Work out the finished part from the listing and answer in its coordinate system (mm). Face numbers are marked on the shaded views. A direction names the side the tool comes from. Give positions to 0.01 mm unless a question says otherwise; leave off trailing zeros. Order: outer loops, then holes, each group sorted by start corner. A loop starts at its lowest first (then second) coordinate and runs counter-clockwise, first axis right, second up. Notation, with made-up numbers: M -35.5,72.5 L -0.5,72.5 A25 cw -0.5,88.5 Z; hole C 74,-23 d9. An arc over 180 degrees is marked long. One line per item, written item: value.
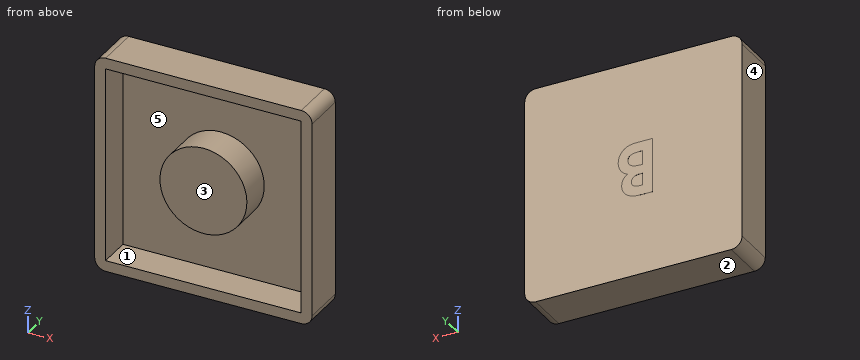
from build123d import *

# Parameters (mm, degrees)
SKETCH1_W           = 12.7
SKETCH1_H           = 12.7
BOSS_EXTRUDE1_DEPTH = 2.54
FILLET1_R           = 0.635
SHELL1_START        = 0.635
SHELL1_OUTLINE_W    = 1.905
SHELL1_OUTLINE_H    = 11.43
SHELL1_DEPTH        = 11.43
SKETCH2_R           = 2.54
BOSS_EXTRUDE2_DEPTH = 1.905
BOSS_EXTRUDE3_DEPTH = 0.00254


# Read off the part's stored shape, not the designer's step: Shell1
with BuildPart() as part:
    # Sketch1 → Boss-Extrude1 (new body)
    with BuildSketch(Plane(origin=(0, 0, 0), x_dir=(1, 0, 0), z_dir=(0, 1, 0))):
        with Locations((6.35, 6.35)):
            Rectangle(SKETCH1_W, SKETCH1_H)
    extrude(amount=BOSS_EXTRUDE1_DEPTH)

    # Fillet1
    fillet1_edges = [part.edges().sort_by_distance(p)[0] for p in [
        (0, 1.27, -12.7),
        (12.7, 1.27, -12.7),
        (12.7, 1.27, 0),
        (0, 1.27, 0),
    ]]
    fillet(fillet1_edges, radius=FILLET1_R)

    # Shell1 outline → Shell1 (cut)
    with BuildSketch(Plane.YZ.offset(SHELL1_START)):
        with Locations((0.9525, -6.35)):
            Rectangle(SHELL1_OUTLINE_W, SHELL1_OUTLINE_H)
    extrude(amount=SHELL1_DEPTH, mode=Mode.SUBTRACT)

    # Sketch2 → Boss-Extrude2 (add)
    with BuildSketch(Plane(origin=(0, 1.905, 0), x_dir=(-1, 0, 0), z_dir=(0, -1, 0))):
        with Locations(Location((-6.35, 6.35, 0), (0, 0, 270))):
            Circle(SKETCH2_R)
    extrude(amount=BOSS_EXTRUDE2_DEPTH)

    # Sketch3 → Boss-Extrude3 (add)
    with BuildSketch(Plane(origin=(0, 2.54, 0), x_dir=(1, 0, 0), z_dir=(0, 1, 0))):
        with BuildLine():
            Line((5.243146154, 4.826), (5.243146154, 8.001))
            Line((5.243146154, 8.001), (5.751960256, 8.001))
            add(Edge.make_bspline(
                [(5.751960256, 8.001), (5.787580425, 8.001004065), (5.856504776, 8.001011931), (5.955944627, 7.99751993), (6.048166691, 7.993002635), (6.132877481, 7.987948833), (6.210221182, 7.979240122), (6.280080178, 7.970062092), (6.34259405, 7.958993954), (6.381242981, 7.94906549), (6.399426202, 7.944394431)],
                knots=[0, 0, 0, 0, 1.311965854, 2.538629056, 3.664479157, 4.713267157, 5.663616078, 6.530575999, 7.308677837, 8, 8, 8, 8], degree=3))
            add(Edge.make_bspline(
                [(6.399426202, 7.944394431), (6.423302618, 7.937805819), (6.470155811, 7.924876846), (6.537264535, 7.898766227), (6.600926521, 7.869742423), (6.661064039, 7.836631691), (6.717307821, 7.799034291), (6.769444122, 7.75665184), (6.818597392, 7.711185567), (6.863022312, 7.66136834), (6.903175119, 7.608727211), (6.93806071, 7.553275975), (6.968371817, 7.495862516), (6.992628642, 7.435764324), (7.010905704, 7.373258168), (7.02427347, 7.308610959), (7.032937594, 7.241618137), (7.03375624, 7.19604073), (7.034171795, 7.172905048)],
                knots=[0, 0, 0, 0, 1.099996261, 2.158545794, 3.195537121, 4.207578794, 5.205712374, 6.197378256, 7.190519799, 8.17788031, 9.159561366, 10.129234751, 11.085776129, 12.040971148, 13.00380137, 13.975669004, 14.972423361, 16, 16, 16, 16], degree=3))
            add(Edge.make_bspline(
                [(7.034171795, 7.172905048), (7.033085241, 7.143181769), (7.030946494, 7.084675147), (7.01728403, 6.998739505), (6.99166478, 6.917517971), (6.958142616, 6.839513663), (6.912562953, 6.765017538), (6.854685596, 6.694065017), (6.785447969, 6.624471365), (6.732338887, 6.582754665), (6.704714663, 6.56105609)],
                knots=[0, 0, 0, 0, 0.986156485, 1.941127874, 2.875419072, 3.804401753, 4.751181392, 5.761612777, 6.835722519, 8, 8, 8, 8], degree=3))
            add(Edge.make_bspline(
                [(6.704714663, 6.56105609), (6.727100009, 6.549628565), (6.770991478, 6.527222351), (6.833304469, 6.490393223), (6.890999497, 6.451220775), (6.944335248, 6.410493172), (6.992192945, 6.366483912), (7.036548712, 6.321728868), (7.075214265, 6.273663764), (7.109790168, 6.22400173), (7.139842981, 6.172023655), (7.166015667, 6.117817318), (7.188122796, 6.061197538), (7.206843685, 6.002452465), (7.220805729, 5.941380042), (7.229909278, 5.877958428), (7.236879525, 5.812403923), (7.237421744, 5.76774983), (7.237697436, 5.745045473)],
                knots=[0, 0, 0, 0, 1.164658916, 2.283573913, 3.35186032, 4.395461096, 5.390182219, 6.362969632, 7.312859996, 8.245001507, 9.165155236, 10.092416118, 11.032087915, 11.979892451, 12.947605196, 13.931445124, 14.948243989, 16, 16, 16, 16], degree=3))
            add(Edge.make_bspline(
                [(7.237697436, 5.745045473), (7.235908383, 5.701681448), (7.232377694, 5.616102718), (7.20656302, 5.490453489), (7.161808578, 5.371326623), (7.101712592, 5.259195582), (7.027662773, 5.157306375), (6.942526717, 5.068052315), (6.847161548, 4.992500734), (6.759175654, 4.941509278), (6.683074784, 4.907289243), (6.620041855, 4.886132259), (6.552345826, 4.866532461), (6.478746667, 4.852769079), (6.400578631, 4.840171317), (6.317079575, 4.832393198), (6.228405558, 4.827122159), (6.167500409, 4.826381615), (6.136114904, 4.826)],
                knots=[0, 0, 0, 0, 1.284142165, 2.534249414, 3.780121997, 5.041676246, 6.291546858, 7.49970053, 8.684500223, 9.883330709, 10.50184324, 11.153274765, 11.851151195, 12.587658647, 13.369265475, 14.195992086, 15.070362669, 16, 16, 16, 16], degree=3))
            Line((6.136114904, 4.826), (5.243146154, 4.826))
        make_face()
        with BuildLine():
            Line((5.813017949, 7.431128205), (5.813017949, 6.739141026))
            Line((5.813017949, 6.739141026), (5.964390144, 6.739141026))
            add(Edge.make_bspline(
                [(5.964390144, 6.739141026), (5.984962986, 6.739320429), (6.024677611, 6.739666755), (6.082041174, 6.744127321), (6.135380025, 6.751737323), (6.184491859, 6.762355191), (6.229834171, 6.775838335), (6.271117303, 6.792061461), (6.308159738, 6.811855437), (6.351194481, 6.841339439), (6.396685308, 6.884726468), (6.436730371, 6.94740802), (6.460316645, 7.019491567), (6.46294352, 7.070330466), (6.4643, 7.096582933)],
                knots=[0, 0, 0, 0, 1.065314748, 2.056525647, 2.977365736, 3.853934255, 4.656397591, 5.425096493, 6.14721249, 6.826394842, 8.123232004, 9.372140726, 10.643011755, 12, 12, 12, 12], degree=3))
            add(Edge.make_bspline(
                [(6.4643, 7.096582933), (6.463214568, 7.12117273), (6.461115928, 7.168716114), (6.437367582, 7.235471259), (6.400481706, 7.29462998), (6.356932744, 7.335119286), (6.315922935, 7.362772289), (6.280807819, 7.380980614), (6.242266343, 7.39728052), (6.199552384, 7.409743825), (6.152909864, 7.419095851), (6.10256535, 7.425963794), (6.048431981, 7.430638408), (6.011041948, 7.430961437), (5.991738902, 7.431128205)],
                knots=[0, 0, 0, 0, 1.347982417, 2.606269829, 3.849316587, 5.153353503, 5.842674298, 6.568177932, 7.326619318, 8.142485038, 9.012069166, 9.942760135, 10.937925643, 12, 12, 12, 12], degree=3))
            Line((5.991738902, 7.431128205), (5.813017949, 7.431128205))
        make_face(mode=Mode.SUBTRACT)
        with BuildLine():
            Line((5.813017949, 6.209974359), (5.813017949, 5.395871795))
            Line((5.813017949, 5.395871795), (5.977110497, 5.395871795))
            add(Edge.make_bspline(
                [(5.977110497, 5.395871795), (6.009551802, 5.396057131), (6.071924261, 5.396413462), (6.161272697, 5.400718795), (6.242512762, 5.408478398), (6.315429202, 5.418165637), (6.3801337, 5.431290331), (6.436407542, 5.447976697), (6.485022448, 5.466334606), (6.525686923, 5.489008804), (6.558907469, 5.515395947), (6.588885529, 5.542364242), (6.613327771, 5.573474717), (6.632666929, 5.607391887), (6.649404936, 5.643273225), (6.65950012, 5.682519883), (6.667186238, 5.723968686), (6.667609226, 5.752637926), (6.667825641, 5.76730609)],
                knots=[0, 0, 0, 0, 1.753078804, 3.370512758, 4.83203934, 6.162291463, 7.344201807, 8.395507345, 9.331626367, 10.147333109, 10.898971645, 11.62040215, 12.321813352, 13.025280112, 13.727906689, 14.453419512, 15.208716525, 16, 16, 16, 16], degree=3))
            add(Edge.make_bspline(
                [(6.667825641, 5.76730609), (6.667348384, 5.784079366), (6.666418815, 5.816749196), (6.658827018, 5.864499638), (6.645030243, 5.909077845), (6.627652532, 5.95162374), (6.603470524, 5.990614032), (6.574731033, 6.027398029), (6.540006391, 6.060730109), (6.500956506, 6.092626322), (6.455408681, 6.120553184), (6.403341547, 6.144784684), (6.344472246, 6.165021941), (6.278618424, 6.181134857), (6.206068781, 6.194809667), (6.126293782, 6.202975038), (6.039957822, 6.209047983), (5.980091063, 6.209658551), (5.949125721, 6.209974359)],
                knots=[0, 0, 0, 0, 0.845221588, 1.646264278, 2.427170338, 3.19324141, 3.95557735, 4.731569926, 5.540061037, 6.376114724, 7.268642756, 8.224665384, 9.265483498, 10.400594375, 11.639216012, 12.983232105, 14.439614077, 16, 16, 16, 16], degree=3))
            Line((5.949125721, 6.209974359), (5.813017949, 6.209974359))
        make_face(mode=Mode.SUBTRACT)
    extrude(amount=BOSS_EXTRUDE3_DEPTH)


solid = part.part
(1) Section B-B, the plane z = -9.75 is taken. Give the vertices of the cut face in (x, y) (3 decimals), then the cut area to 3 significant figures.
Findings:
outline: M 0,0 L 0.635,0 L 0.635,1.905 L 12.065,1.905 L 12.065,0 L 12.7,0 L 12.7,2.54 L 0,2.54 Z
area: 10.5 mm^2
(2) Find the intervals of material crossed by probe 1 along Z at (x, y) = (6.5, 0.55) (3 decimals); probe 2 along Z at (x, y) = (11, 1.2) (3 decimals); probe 3 along X at (y, z) = (0.8, -5) (3 decimals), in increasing order. Write a range as from..to.
Findings:
probe 1: z = -12.7..-12.065, -8.886..-3.814, -0.635..0
probe 2: z = -12.7..-12.065, -0.635..0
probe 3: x = 0..0.635, 4.198..8.502, 12.065..12.7
(3) Section C-C, the plane x = 2.25 is taken. Give the vertices of the cut face in (y, z) (3 decimals), then the cut area to 3 significant figures.
Findings:
outline: M 0,-12.7 L 2.54,-12.7 L 2.54,0 L 0,0 L 0,-0.635 L 1.905,-0.635 L 1.905,-12.065 L 0,-12.065 Z
area: 10.5 mm^2
(4) Section D-D, the plane x = 4.25 is taken. Give the vertices of the cut face in (y, z) (3 decimals), then the cut area to 3 significant figures.
Findings:
outline: M 0,-12.7 L 2.54,-12.7 L 2.54,0 L 0,0 L 0,-0.635 L 1.905,-0.635 L 1.905,-4.921 L 0,-4.921 L 0,-7.779 L 1.905,-7.779 L 1.905,-12.065 L 0,-12.065 Z
area: 15.9 mm^2
(5) Section A-A, the plane y = 1.1 is taken. Give the vertices of the cut face in (x, z) (3 decimals), then the cut area to 3 significant figures.
Findings:
outline: M 0,-12.065 A0.635 ccw 0.635,-12.7 L 12.065,-12.7 A0.635 ccw 12.7,-12.065 L 12.7,-0.635 A0.635 ccw 12.065,0 L 0.635,0 A0.635 ccw 0,-0.635 Z; C 6.35,-6.35 d5.08; hole M 0.635,-12.065 L 12.065,-12.065 L 12.065,-0.635 L 0.635,-0.635 Z
area: 50.6 mm^2
(6) Which of the six approach directions +Z, -Z, +X, -X, +Y, -Y give full straight-line access (tool end or side, diameter ignored) to the marked faces 4 and 5?
Findings:
face 4: +Z, -Z, -X, +Y, -Y
face 5: -Y
(7) Determine the mould class of the marked faces 1, 2 and 3 for opening direction Z: pulls with the +Z half, pulls with the -Z half, needs draft (parallel to the pull), parting line crosses it, or undercut.
Findings:
face 1: undercut
face 2: pulls with the -Z half
face 3: needs draft
